```python
from build123d import *

# Parameters (mm, degrees)
SKETCH1_R           = 10
BOSS_EXTRUDE1_DEPTH = 50
SKETCH2_W           = 44.116747391
SKETCH2_H           = 26
CUT_EXTRUDE1_DEPTH  = 50
SKETCH3_R           = 10
CUT_EXTRUDE2_DEPTH  = 50
CUT_EXTRUDE3_DEPTH  = 36
CUT_EXTRUDE4_DEPTH  = 50
FILLET1_R           = 10
SKETCH6_W           = 2.5
SKETCH6_H           = 26
CUT_EXTRUDE5_DEPTH  = 50


with BuildPart() as part:
    # Sketch1 → Boss-Extrude1 (new body)
    with BuildSketch(Plane(origin=(0, 0, 0), x_dir=(1, 0, 0), z_dir=(0, 1, 0))):
        with BuildLine():
            Line((0, 18), (50, 18))
            Line((50, 18), (50, -18))
            Line((50, -18), (0, -18))
            ThreePointArc((0, -18), (-18, 0), (0, 18))
        make_face()
        Circle(SKETCH1_R, mode=Mode.SUBTRACT)
    extrude(amount=BOSS_EXTRUDE1_DEPTH)

    # Sketch2 → Cut-Extrude1 (cut)
    with BuildSketch(Plane(origin=(0, 0, -18), x_dir=(-1, 0, 0), z_dir=(0, 0, -1))):
        with Locations((2.058373696, 25)):
            Rectangle(SKETCH2_W, SKETCH2_H)
    extrude(amount=-CUT_EXTRUDE1_DEPTH, mode=Mode.SUBTRACT)

    # Sketch3 → Cut-Extrude2 (cut)
    with BuildSketch(Plane(origin=(0, 0, -18), x_dir=(-1, 0, 0), z_dir=(0, 0, -1))):
        with Locations((-35, 25)):
            Circle(SKETCH3_R)
    extrude(amount=-CUT_EXTRUDE2_DEPTH, mode=Mode.SUBTRACT)

    # Sketch4 → Cut-Extrude3 (cut)
    with BuildSketch(Plane(origin=(0, 0, -18), x_dir=(-1, 0, 0), z_dir=(0, 0, -1))):
        Polygon((-15, 0), (-25, 7), (-50, 7), (-50, 0), align=None)
        Polygon((-50, 50), (-50, 43), (-25, 43), (-15, 50), align=None)
    extrude(amount=-CUT_EXTRUDE3_DEPTH, mode=Mode.SUBTRACT)

    # Sketch5 → Cut-Extrude4 (cut)
    with BuildSketch(Plane(origin=(0, 50, 0), x_dir=(1, 0, 0), z_dir=(0, 1, 0))):
        Polygon((15, 18), (25, 13), (50, 13), (50, 18), align=None)
        Polygon((15, -18), (25, -13), (50, -13), (50, -18), align=None)
    extrude(amount=-CUT_EXTRUDE4_DEPTH, mode=Mode.SUBTRACT)

    # Fillet1
    fillet1_edges = [part.edges().sort_by_distance(p)[0] for p in [
        (50, 7, 0),
        (50, 43, 0),
    ]]
    fillet(fillet1_edges, radius=FILLET1_R)

    # Sketch6 → Cut-Extrude5 (cut)
    with BuildSketch(Plane.ZY.offset(-20)):
        with Locations((-14.25, 25)):
            Rectangle(SKETCH6_W, SKETCH6_H)
        with Locations((14.25, 25)):
            Rectangle(SKETCH6_W, SKETCH6_H)
    extrude(amount=-CUT_EXTRUDE5_DEPTH, mode=Mode.SUBTRACT)


solid = part.part
```
CAD build for the part. Positions are in the model's coordinates, mm. A direction names the side the tool comes from. Coordinates: 2 decimals unless noted, no trailing zeros. Order: outer loops, then holes, each group sorted by start corner. A loop starts at its lowest first (then second) coordinate and runs counter-clockwise, first axis right, second up. Notation, with made-up numbers: (-9, -15.5) - (42, -15.5) arc R27 ccw to (42, 19.5) - close; hole circle Ø8 at (25.25, 15.25). An arc over 180 degrees is marked (long way). Answer in a Markdown table with one row per item.
1. Slice it at D-D, the plane x = 6. List the corners of the cut face in (y, z).
Answer:
| item | result |
|---|---|
| outline | (0, -18) - (12, -18) - (12, -8) - (0, -8) - close; (0, 8) - (12, 8) - (12, 18) - (0, 18) - close; (38, -18) - (50, -18) - (50, -8) - (38, -8) - close; (38, 8) - (50, 8) - (50, 18) - (38, 18) - close |
2. Flat gauge pins, fed straight in: P1, Ø1.5, axis at x = 18, z = -12.5, coming from the -Y side (3 decimals); P2, Ø5, axis at x = 18.5, y = 24.5, coming from the -Z side; P3, Ø4.5, axis at x = 33, z = -5, coming from the +Y side; P4, Ø12, axis at x = 0, z = 0, coming from the +Y side. Where does each tip first touch, or does it go through?
Answer:
| item | result |
|---|---|
| P1 | y = 1.575 |
| P2 | z = -13 |
| P3 | y = 43 |
| P4 | through |
3. Drill centre lines: L1, parallel to Y at x = -13.5, z = 9; L2, parallel to X at y = 25.5, z = -8; L3, parallel to X at y = 30, z = 9.5. Where is each one in solid material? Low to high. Write a range as from..to.
Answer:
| item | result |
|---|---|
| L1 | 0..12, 38..50 |
| L2 | 20..25.01, 44.99..50 |
| L3 | 20..26.34, 43.66..50 |
4. Slice it at C-C, the plane x = 35. List the corners of the cut face in (y, z).
Answer:
| item | result |
|---|---|
| outline | (7, -13) - (15, -13) - (15, 13) - (7, 13) - close; (35, -13) - (43, -13) - (43, 13) - (35, 13) - close |
5. Slice it at B-B, the plane z = 0. List the corners of the cut face in (x, y), then the cut area to 3 significant figures.
Answer:
| item | result |
|---|---|
| outline | (-18, 0) - (-10, 0) - (-10, 12) - (-18, 12) - close; (-18, 38) - (-10, 38) - (-10, 50) - (-18, 50) - close; (10, 0) - (15, 0) - (25, 7) - (40, 7) arc R10 ccw to (50, 17) - (50, 33) arc R10 ccw to (40, 43) - (25, 43) - (15, 50) - (10, 50) - (10, 38) - (20, 38) - (20, 12) - (10, 12) - close; hole circle Ø20 at (35, 25) |
| area | 1,150 mm² |
6. Pull direction X, two halves, no side cores. Call faces 1 (the face through (42.37, 31.76, -0.18)), 2 (the face through (19, 43, -16)), 3 (the face through (-18, 44, 0)), 4 (the face through (33, 43, 0)): +X half, -X half, draft (parallel to the pull), parting line (faces both ways), or undercut.
Answer:
| item | result |
|---|---|
| face 1 | undercut |
| face 2 | +X half |
| face 3 | -X half |
| face 4 | draft |
7. 3-axis set-ups, long thin cutter, end or side, ignore diameter. For faces 5 (the face through (20, 25, 0)), 6 (the face through (24.8, 25.3, 13)), 7 (the face through (20.07, 46.45, -0.25)): which of +Z, -Z, +X, -X, +Y, -Y reach the whole face in a straight line?
Answer:
| item | result |
|---|---|
| face 5 | +Z, -Z, -X |
| face 6 | +Z, +X |
| face 7 | +Z, -Z, +X, +Y |
8. Slice it at A-A, the plane y = 25. List the corners of the cut face in (x, z).
Answer:
| item | result |
|---|---|
| outline | (20, -13) - (25, -13) - (25, 13) - (20, 13) - close; (45, -13) - (50, -13) - (50, 13) - (45, 13) - close |
